Check sheet for the modelled part. Datum: model origin and axes. Units: mm. A direction names the side the tool comes from. Coordinates: 2 decimals unless noted, no trailing zeros. Write each loop counter-clockwise with the first axis right and the second up, starting at its lowest first coordinate (ties: lowest second). Pieces come first, ordered by that corner, then holes. Notation, with made-up numbers: (44.25, -11) -> (82.25, -11) arc R21 cw to (82.25, 6) -> close; hole circle Ø9 at (17.5, 28). An arc over 180 degrees is marked (long way). One line per item, written item: value. Start each with the question number.
1) Sectioned sample at C-C on y = 1.3. Give the number of separate pieces and of enclosed holes in the cut face, plus the area to 3 significant figures.
2) Scan lines: line 1 along X through (y, z) = (3.1, 2); line 2 along X through (y, z) = (4.6, 1.5); line 3 along Z through (x, y) = (38.5, 4.4). Record each from-to range of solid material in increasing order. Write a range as [from, to].
3) Sectioned sample at D-D on x = 26. Enter the section's corners in (y, z), plus the area to 3 significant figures.
4) Set-up check for faces 1 (the flat face through (-8.965, 2.465, 26.528)), 2 (the flat face through (47, 2, -12)), 3 (the cylindrical face through (71.53, 2.54, 33.06)), 4 (the flat face through (51, 2, 51)), 5 (the flat face through (-18.342, 2.465, 20.769)): record each of +Z, -Z, +X, -X, +Y, -Y from which the full face is reachable in a straight line by a thin tool's end or side.
5) Sectioned sample at B-B on x = -19. Enter the section's corners in (y, z).
6) Gauge pin test, flat ends, axial feed: P1, Ø2, axis at x = 33, y = 1, coming from the -Z side; P2, Ø2.5, axis at x = 27.5, y = 1.5, coming from the +Z side; P3, Ø1, axis at y = 2, z = -22, coming from the +X side; P4, Ø4, axis at x = -19, z = 32.91, coming from the +Y side. Record the tip position at first contact, or that the pin passes through.
7) Sectioned sample at A-A on x = 38. Enter the section's corners in (y, z) (3 decimals).
```python
from build123d import *

# Parameters (mm, degrees)
SKETCH1_R               = 17.5
SKETCH1_R_2             = 9
BOSS_EXTRUDE1_DEPTH     = 5
BOSS_EXTRUDE3_DEPTH     = 5
SKETCH6_W               = 47.262260797
SKETCH6_H               = 24
BOSS_EXTRUDE4_DEPTH     = 5
SKETCH4_R               = 3.125
CUT_EXTRUDE1_DEPTH      = 63.69968102
CIRPATTERN1_COUNT       = 3
BOSS_EXTRUDE5_DEPTH     = 5
CUT_EXTRUDE_THIN1_DEPTH = 10
FILLET1_R               = 1.2
FILLET2_R               = 5


with BuildPart() as part:
    # Sketch1 → Boss-Extrude1 (new body)
    with BuildSketch(Plane(origin=(0, 0, 0), x_dir=(1, 0, 0), z_dir=(0, 1, 0))):
        with Locations(Location((0, 0, 0), (0, 0, 270))):
            Circle(SKETCH1_R)
        with Locations(Location((0, 0, 0), (0, 0, 270))):
            Circle(SKETCH1_R_2, mode=Mode.SUBTRACT)
    extrude(amount=BOSS_EXTRUDE1_DEPTH)

    # Sketch3 → Boss-Extrude3 (add)
    with BuildSketch(Plane(origin=(0, 0, 0), x_dir=(1, 0, 0), z_dir=(0, 1, 0))):
        with BuildLine():
            Line((38, 5.5), (10.009906254, 5.5))
            Line((10.009906254, 5.5), (10.009906254, -5.5))
            Line((10.009906254, -5.5), (38, -5.5))
            ThreePointArc((38, -5.5), (32.5, 0), (38, 5.5))
        make_face()
        with BuildLine():
            ThreePointArc((43.5, 0), (41.889087297, 3.889087297), (38, 5.5))
            Line((38, 5.5), (38, -5.5))
            ThreePointArc((38, -5.5), (41.889087297, -3.889087297), (43.5, 0))
        make_face()
        with BuildLine():
            Line((38, -5.5), (38, 5.5))
            ThreePointArc((38, 5.5), (32.5, 0), (38, -5.5))
        make_face()
    boss_extrude3 = extrude(amount=BOSS_EXTRUDE3_DEPTH)

    # Sketch6 → Boss-Extrude4 (add)
    with BuildSketch(Plane(origin=(0, 0, 0), x_dir=(1, 0, 0), z_dir=(0, 1, 0))):
        with Locations((36.368869602, 0)):
            Rectangle(SKETCH6_W, SKETCH6_H)
    extrude(amount=BOSS_EXTRUDE4_DEPTH)

    # Sketch4 → Cut-Extrude1 (cut, symmetric)
    with BuildSketch(Plane(origin=(0, 5, 0), x_dir=(1, 0, 0), z_dir=(0, 1, 0))):
        with Locations(Location((38, 0, 0), (0, 0, 270))):
            Circle(SKETCH4_R)
    cut_extrude1 = extrude(amount=CUT_EXTRUDE1_DEPTH, both=True, mode=Mode.SUBTRACT)

    # CirPattern1: Boss-Extrude3, Cut-Extrude1 ×3 about axis
    cirpattern1_axis = Axis((0, 0, 0), (0, 1, 0))
    add([boss_extrude3.rotate(cirpattern1_axis, i * 360 / CIRPATTERN1_COUNT) for i in range(1, CIRPATTERN1_COUNT)])
    add([cut_extrude1.rotate(cirpattern1_axis, i * 360 / CIRPATTERN1_COUNT) for i in range(1, CIRPATTERN1_COUNT)], mode=Mode.SUBTRACT)

    # Sketch7 → Boss-Extrude5 (add)
    with BuildSketch(Plane(origin=(0, 0, 0), x_dir=(1, 0, 0), z_dir=(0, 1, 0))):
        with BuildLine():
            Line((42.426406871, -42.426406871), (60.104076401, -60.104076401))
            ThreePointArc((60.104076401, -60.104076401), (78.529760263, -32.528091751), (85, 0))
            ThreePointArc((85, 0), (84.786902365, 6.015079992), (84.148677946, 12))
            Line((84.148677946, 12), (58.787753827, 12))
            ThreePointArc((58.787753827, 12), (59.69616918, 6.03053772), (60, 0))
            ThreePointArc((60, 0), (55.432771951, -22.961005942), (42.426406871, -42.426406871))
        make_face()
    extrude(amount=BOSS_EXTRUDE5_DEPTH)

    # Sketch8 → Cut-Extrude-Thin1 (cut)
    with BuildSketch(Plane(origin=(0, 5, 0), x_dir=(1, 0, 0), z_dir=(0, 1, 0))):
        with BuildLine():
            ThreePointArc((77.602850937, -13.6834764), (71.417053618, -33.302319025), (60.364302118, -50.651663643))
            Line((60.364302118, -50.651663643), (62.202808781, -52.194353907))
            ThreePointArc((62.202808781, -52.194353907), (73.592192307, -34.316602853), (79.966389545, -14.100232027))
            Line((79.966389545, -14.100232027), (77.602850937, -13.6834764))
        make_face()
        with BuildLine():
            ThreePointArc((68.247177284, -12.033818712), (62.807129642, -29.287445539), (53.086879908, -44.545181351))
            Line((53.086879908, -44.545181351), (54.925386572, -46.087871615))
            ThreePointArc((54.925386572, -46.087871615), (64.982268331, -30.301729367), (70.610715891, -12.450574339))
            Line((70.610715891, -12.450574339), (68.247177284, -12.033818712))
        make_face()
    extrude(amount=-CUT_EXTRUDE_THIN1_DEPTH, mode=Mode.SUBTRACT)

    # Fillet1
    fillet1_edges = [part.edges().sort_by_distance(p)[0] for p in [
        (70.610715891, 2.5, 12.450574339),
        (79.966389545, 2.5, 14.100232027),
        (77.602850937, 2.5, 13.6834764),
        (68.247177284, 2.5, 12.033818712),
        (62.202808781, 2.5, 52.194353907),
        (60.364302118, 2.5, 50.651663643),
        (54.925386572, 2.5, 46.087871615),
        (53.086879908, 2.5, 44.545181351),
    ]]
    fillet(fillet1_edges, radius=FILLET1_R - 0.0001)  # a hair under: the kernel refuses the full size

    # Fillet2
    fillet2_edges = [part.edges().sort_by_distance(p)[0] for p in [
        (84.148677946, 2.5, -12),
        (58.787753827, 2.5, 12),
        (42.426406871, 2.5, 42.426406871),
        (60.104076401, 2.5, 60.104076401),
    ]]
    fillet(fillet2_edges, radius=FILLET2_R)


solid = part.part
```
Answers:
1. separate pieces: 1
1. enclosed holes: 6
1. area: 3,750 mm2
2. line 1: x = [-17.39, -8.77], [8.77, 35.6], [40.4, 84.98]
2. line 2: x = [-17.44, -8.87], [8.87, 35.26], [40.74, 84.99]
2. line 3: z = [-12, -3.08], [3.08, 12]
3. outline: (0, -12) -> (5, -12) -> (5, 12) -> (0, 12) -> close
3. area: 120 mm2
4. face 1: +Z, +Y, -Y
4. face 2: -Z, +X, +Y, -Y
4. face 3: +Y, -Y
4. face 4: +Z, -X, +Y, -Y
4. face 5: -X, +Y, -Y
5. outline: (0, -38.41) -> (5, -38.41) -> (5, -36.03) -> (0, -36.03) -> close; (0, -29.78) -> (5, -29.78) -> (5, -21.91) -> (0, -21.91) -> close; (0, 21.91) -> (5, 21.91) -> (5, 29.78) -> (0, 29.78) -> close; (0, 36.03) -> (5, 36.03) -> (5, 38.41) -> (0, 38.41) -> close
6. P1: stops at z = -12
6. P2: stops at z = 12
6. P3: stops at x = -6.06
6. P4: passes through
7. outline: (0, -12) -> (5, -12) -> (5, -3.125) -> (0, -3.125) -> close; (0, 3.125) -> (5, 3.125) -> (5, 12) -> (0, 12) -> close
